Could you check a few things on this model? Use its own coordinates, in mm. A direction names the side the tool comes from. Give positions to 0.01 mm unless a question says otherwise; leave off trailing zeros. Write each loop counter-clockwise with the first axis right and the second up, starting at its lowest first coordinate (ties: lowest second). Pieces come first, ordered by that corner, then holes. Notation, with made-up numbers: (87.25, 28) -> (108.25, 28) arc R16 cw to (108.25, 42) -> close; hole circle Ø4 at (67.5, 60). An arc over 180 degrees is marked (long way). One line per question, with ' | ' between items.
from build123d import *

# Parameters (mm, degrees)
SKETCH1_R                    = 14.5
BOSS_EXTRUDE1_DEPTH          = 20
CUT_EXTRUDE1_DEPTH           = 49.928519291
CUT_EXTRUDE1_DEPTH_BACK      = 49.928519291
SKETCH2_R                    = 3
CUT_EXTRUDE_THIN1_DEPTH      = 49.928519332
CUT_EXTRUDE_THIN1_DEPTH_BACK = 49.928519332
SKETCH5_R                    = 40
SKETCH5_R_2                  = 30


with BuildPart() as part:
    # Sketch1 → Boss-Extrude1 (new, symmetric)
    with BuildSketch(Plane(origin=(0, 0, 0), x_dir=(1, 0, 0), z_dir=(0, 1, 0))):
        with BuildLine():
            Line((-25, 21.5), (-25, 13.5))
            Line((-25, 13.5), (-21.5, 13.5))
            ThreePointArc((-21.5, 13.5), (-17.257359313, 11.742640687), (-15.5, 7.5))
            Line((-15.5, 7.5), (-15.5, 0))
            ThreePointArc((-15.5, 0), (0, -15.5), (15.5, 0))
            Line((15.5, 0), (15.5, 7.5))
            ThreePointArc((15.5, 7.5), (17.257359313, 11.742640687), (21.5, 13.5))
            Line((21.5, 13.5), (25, 13.5))
            Line((25, 13.5), (25, 21.5))
            Line((25, 21.5), (-25, 21.5))
        make_face()
        with Locations(Location((0, 0, 0), (0, 0, 270))):
            Circle(SKETCH1_R, mode=Mode.SUBTRACT)
    extrude(amount=BOSS_EXTRUDE1_DEPTH, both=True)

    # Sketch2 → Cut-Extrude1 (cut, two sides: drawn at the far end of the back side and taken through both)
    with BuildSketch(Plane(origin=(0, 0, -21.5), x_dir=(-1, 0, 0), z_dir=(0, 0, -1)).offset(-CUT_EXTRUDE1_DEPTH_BACK)):
        with Locations(Location((-20, 15, 0), (0, 0, 120))):
            Circle(SKETCH2_R)
        with Locations(Location((20, 15, 0), (0, 0, 60))):
            Circle(SKETCH2_R)
        with Locations(Location((20, -15, 0), (0, 0, 60))):
            Circle(SKETCH2_R)
        with Locations(Location((-20, -15, 0), (0, 0, 120))):
            Circle(SKETCH2_R)
    extrude(amount=CUT_EXTRUDE1_DEPTH + CUT_EXTRUDE1_DEPTH_BACK, mode=Mode.SUBTRACT)

    # Sketch5 → Cut-Extrude-Thin1 (cut, two sides: drawn at the far end of the back side and taken through both)
    with BuildSketch(Plane(origin=(0, 0, -21.5), x_dir=(-1, 0, 0), z_dir=(0, 0, -1)).offset(-CUT_EXTRUDE_THIN1_DEPTH_BACK)):
        Circle(SKETCH5_R)
        Circle(SKETCH5_R_2, mode=Mode.SUBTRACT)
    extrude(amount=CUT_EXTRUDE_THIN1_DEPTH + CUT_EXTRUDE_THIN1_DEPTH_BACK, mode=Mode.SUBTRACT)


solid = part.part
Q1. If I drill on line 1 along Y through (x, z) = (-20, -16.75); line 2 along Y through (x, z) = (-18, -17); line 3 along X through (y, z) = (-7, 12), over which ranges is the centre line in solid material (lowest first)?
Answer below:
line 1: y = -20 to -18, -12 to 12, 18 to 20 | line 2: y = -20 to -17.24, -12.76 to 12.76, 17.24 to 20 | line 3: x = -9.81 to -8.14, 8.14 to 9.81
Q2. Imagine slicing it at B-B on x = 0. Please give me the cut outline in (y, z), and give its area (3 significant figures).
Answer below:
outline: (-20, -21.5) -> (20, -21.5) -> (20, -14.5) -> (-20, -14.5) -> close; (-20, 14.5) -> (20, 14.5) -> (20, 15.5) -> (-20, 15.5) -> close | area: 320 mm^2
Q3. Imagine slicing it at C-C on y = -3. Please give me the cut outline in (x, z), and give its area (3 significant figures).
Answer below:
outline: (-25, -21.5) -> (25, -21.5) -> (25, -13.5) -> (21.5, -13.5) arc R6 cw to (15.5, -7.5) -> (15.5, 0) arc R15.5 ccw to (-15.5, 0) -> (-15.5, -7.5) arc R6 cw to (-21.5, -13.5) -> (-25, -13.5) -> close; hole circle Ø29 at (0, 0) | area: 551 mm^2
Q4. Imagine slicing it at D-D on z = 11. Please give me the cut outline in (x, y), and give its area (3 significant figures).
Answer below:
outline: (-10.92, -20) -> (-9.45, -20) -> (-9.45, 20) -> (-10.92, 20) -> close; (9.45, -20) -> (10.92, -20) -> (10.92, 20) -> (9.45, 20) -> close | area: 118 mm^2
Q5. If we mould it in two halves opening along Y, with no side actions, what happens to faces 4 (the flat face through (15.5, 0, -4)), 5 (the cylindrical face through (-17.23, 16.15, -17.53)), 6 (the flat face through (-2, -20, -15)), 7 (the flat face through (-2, 20, -15))? For each: +Y half, -Y half, draft (parallel to the pull), parting line (faces both ways), or undercut.
Answer below:
face 4: draft | face 5: undercut | face 6: -Y half | face 7: +Y half
Q6. Will these pins go through, and if not, where does the flat tip stop? pin 1 (6 mm diameter, centred on x = 19, y = 3.5, fed in from +Z); pin 2 (4 mm diameter, centred on x = 15.5, y = -4.5, fed in from +Z); pin 3 (2.5 mm diameter, centred on y = -4.5, z = -5, fed in from +X); pin 4 (8 mm diameter, centred on x = -6.5, z = 2, fed in from -Y).
Answer below:
pin 1: stops at z = -9.9 | pin 2: stops at z = 7.62 | pin 3: stops at x = 15.5 | pin 4: passes through
Q7. Imagine slicing it at A-A on y = 15. Please give me the cut outline in (x, z).
Answer below:
outline: (-25, -21.5) -> (-23, -21.5) -> (-23, -13.5) -> (-25, -13.5) -> close; (-17, -21.5) -> (17, -21.5) -> (17, -11.47) arc R6 cw to (15.5, -7.5) -> (15.5, 0) arc R15.5 ccw to (-15.5, 0) -> (-15.5, -7.5) arc R6 cw to (-17, -11.47) -> close; (23, -21.5) -> (25, -21.5) -> (25, -13.5) -> (23, -13.5) -> close; hole circle Ø29 at (0, 0)
Q8. On a 3-axis mill with a long thin cutter (end or side, diameter ignored), from which of +Z, -Z, +X, -X, +Y, -Y can I reach the whole of each face in a straight line? I mean faces 1 (the flat face through (23, 0, -13.5)), 2 (the cylindrical face through (24, -18, -17)), 3 (the flat face through (-23, 0, -13.5)). Say none if no direction works.
Answer below:
face 1: +Z, +X, +Y, -Y | face 2: +Z, -Z, +X, -Y | face 3: +Z, -X, +Y, -Y
